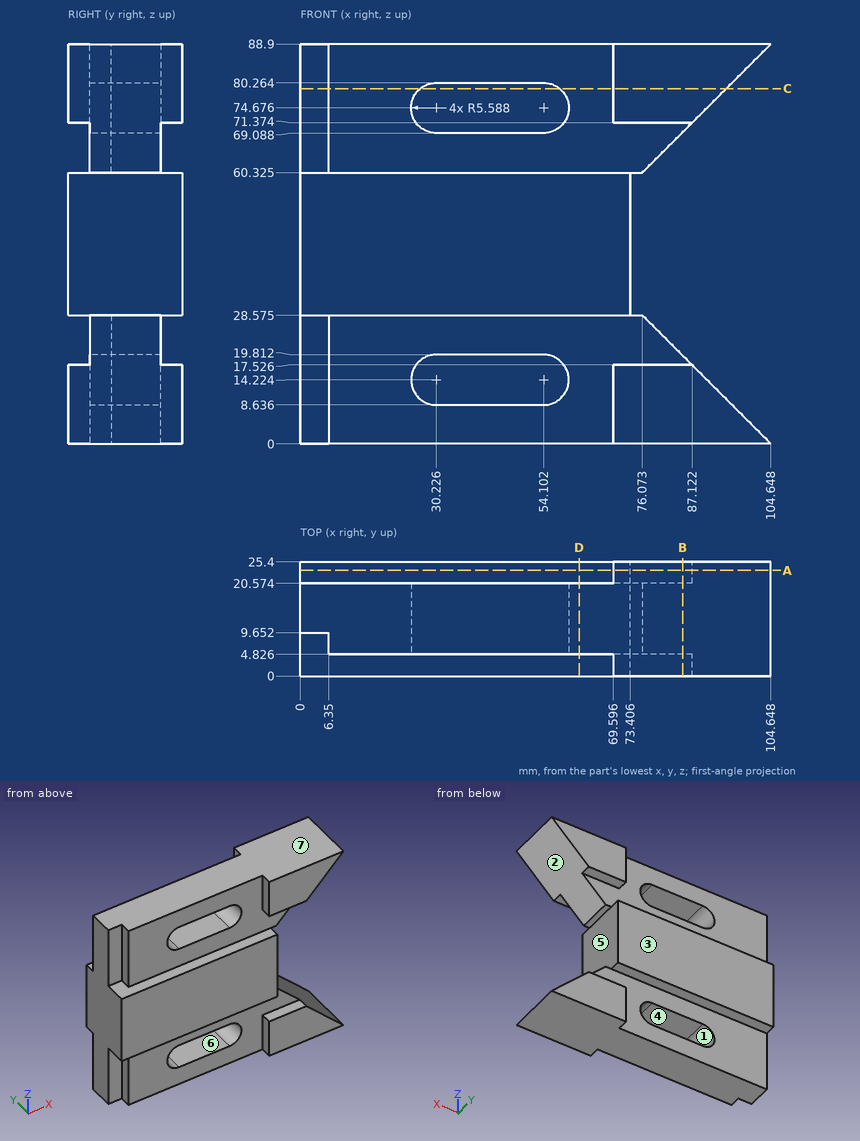
Answer from the drawing. Dimensions are ordinates in mm from the lowest x, y and z of the part. A direction names the side the tool comes from. Give positions to 0.01 mm unless a question says otherwise; leave off trailing zeros. Loops run counter-clockwise (first coordinate to the right, second up) from the corner with the lowest first, then second, coordinate; pieces in that order, holes last. Notation, with made-up numbers: (-36, -29) - (8, -29) arc R27 ccw to (8, 0) - close; hole circle Ø8 at (7, 28). An arc over 180 degrees is marked (long way). Write each question's results on one line, items separated by ' | '.
1. Which of the six approach directions +Z, -Z, +X, -X, +Y, -Y give full straight-line access (tool end or side, diameter ignored) to the marked faces 5, 6 and 7?
Resolved:
face 5: +X, +Y, -Y | face 6: +Y, -Y | face 7: +Z, +X, -X, +Y, -Y
2. For a pull along X with two mould halves and no side action, classify the marked faces 1, 2, 3 and 4 as +X half, -X half, draft (parallel to the pull), parting line (faces both ways), or undercut.
Resolved:
face 1: undercut | face 2: +X half | face 3: draft | face 4: undercut
3. Find section C-C, the plane z = 79. Write down the section's boundary in (x, y).
Resolved:
outline: (0, 9.65) - (6.35, 9.65) - (6.35, 4.83) - (26.69, 4.83) - (26.69, 20.57) - (0, 20.57) - close; (57.64, 4.83) - (69.6, 4.83) - (69.6, 0) - (94.75, 0) - (94.75, 25.4) - (69.6, 25.4) - (69.6, 20.57) - (57.64, 20.57) - close
4. Consider probe 1 along Z at (x, y) = (52, 9.5); probe 2 along Z at (x, y) = (76, 20) (3 decimals); probe 3 along Z at (x, y) = (85.5, 21). Determine where each line is inside the solid, lowest interval first. Write a range as from..to.
Resolved:
probe 1: z = 0..8.64, 19.81..69.09, 80.26..88.9 | probe 2: z = 0..28.575, 60.325..88.9 | probe 3: z = 0..17.53, 71.37..88.9
5. Find section A-A, the plane y = 23.5. Write down the section's boundary in (x, z) (3 decimals).
Resolved:
outline: (0, 28.575) - (73.406, 28.575) - (73.406, 60.325) - (0, 60.325) - close; (69.596, 0) - (104.648, 0) - (87.122, 17.526) - (69.596, 17.526) - close; (69.596, 71.374) - (87.122, 71.374) - (104.648, 88.9) - (69.596, 88.9) - close
6. Flat-ended cylindrical pins translate along their axes: P1, Ø6, axis at x = 74.5, z = 25.5, coming from the +Y side; P2, Ø3, axis at x = 62.5, z = 77, coming from the -Y side; P3, Ø8, axis at x = 45.5, y = 11, coming from the -Z side; P4, Ø2.5, axis at y = 3, z = 5.5, coming from the -X side. Find the tip coordinate at first contact, or state that the pin passes through.
Resolved:
P1: stops at y = 20.57 | P2: stops at y = 4.83 | P3: stops at z = 0 | P4: stops at x = 69.6
7. Find section B-B, the plane x = 85. Write down the section's boundary in (y, z), then the cut area to 3 significant figures.
Resolved:
outline: (0, 0) - (25.4, 0) - (25.4, 17.53) - (20.57, 17.53) - (20.57, 19.65) - (4.83, 19.65) - (4.83, 17.53) - (0, 17.53) - close; (0, 71.37) - (4.83, 71.37) - (4.83, 69.25) - (20.57, 69.25) - (20.57, 71.37) - (25.4, 71.37) - (25.4, 88.9) - (0, 88.9) - close | area: 957 mm^2
8. Find section D-D, the plane x = 62. Write down the section's boundary in (y, z) (3 decimals).
Resolved:
outline: (0, 28.575) - (4.826, 28.575) - (4.826, 0) - (20.574, 0) - (20.574, 28.575) - (25.4, 28.575) - (25.4, 60.325) - (20.574, 60.325) - (20.574, 88.9) - (4.826, 88.9) - (4.826, 60.325) - (0, 60.325) - close
